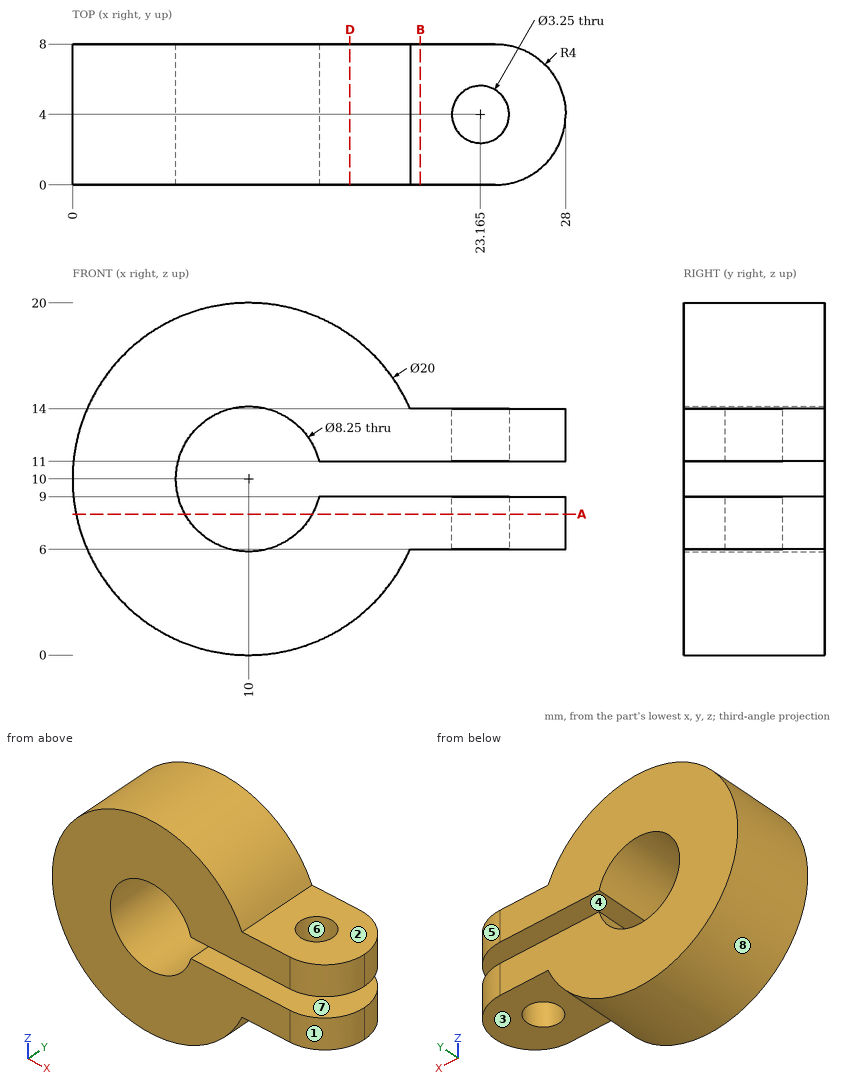
Input: dimensioned drawing with shaded views. Units: mm. Origin: part minimum x, y, z. A direction names the side the tool comes from. Coordinates: 2 decimals unless noted, no trailing zeros. Loops run counter-clockwise (first coordinate to the right, second up) from the corner with the lowest first, then second, coordinate; pieces in that order, holes last. Notation, with made-up numbers: (85, 70) - (90, 70) arc R28 ccw to (90, 91) - close; hole circle Ø1 at (57, 48). An arc over 180 degrees is marked (long way). One line per question, with ' | ' between items. Start each with the question number.
(1) Cut plane D-D on x = 15.75. Output: boundary loops of the cut face in (y, z).
(2) First-contact query: pin 1 (2 mm diameter, centred on y = 6.5, z = 3.5, fed in from +X); pin 2 (4 mm diameter, centred on x = 19, y = 3, fed in from +Z). Flat tips, straight axial feed; report the tip coordinate or a pass-through.
(3) Draft query along X for the marked faces 5, 6, 7 and 8. Return one class per face: +X half, -X half, draft (parallel to the pull), parting line (faces both ways), or undercut.
(4) Cut plane B-B on x = 19.75. Output: boundary loops of the cut face in (y, z).
(5) Cut plane A-A on z = 8. Count the separate pieces of the cut face and the enclosed holes in it, and give its area (4 significant figures).
(6) Ray query, L1, parallel to Z at x = 26.5, y = 1.5; L2, parallel to Y at x = 24.5, z = 12.25; L3, parallel to X at y = 3.5, z = 10 (3 decimals). Return the intervals inside material, ascending. Write a range as from..to.
(7) Reachability of the marked faces 1, 2, 3 and 4 from +Z, -Z, +X, -X, +Y, -Y: full face, straight path, thin tool, end or side. Return the list, or none.
Here are the results:
1) outline: (0, 1.82) - (8, 1.82) - (8, 9) - (0, 9) - close; (0, 11) - (8, 11) - (8, 18.18) - (0, 18.18) - close
2) pin 1: x = 18.35 | pin 2: z = 17.14
3) face 5: +X half | face 6: undercut | face 7: draft | face 8: parting line
4) outline: (0, 6) - (8, 6) - (8, 9) - (0, 9) - close; (0, 11) - (8, 11) - (8, 14) - (0, 14) - close
5) separate pieces: 2 | enclosed holes: 1 | area: 149.5 mm²
6) L1: 6..9, 11..14 | L2: 0.03..3.07, 4.93..7.97 | L3: 0..5.875
7) face 1: +Z, -Z, +X, -Y | face 2: +Z, +X, +Y, -Y | face 3: -Z, +X, +Y, -Y | face 4: +X, +Y, -Y
